```python
from build123d import *

# Parameters (mm, degrees)
SKETCH1_W                = 184.15
SKETCH1_H                = 184.15
BOSS_EXTRUDE1_DEPTH      = 3.175
CUT_EXTRUDE1_DEPTH       = 131.368453815
SKETCH3_R                = 6.477
SKETCH3_R_2              = 2.20345
CUT_EXTRUDE2_DEPTH       = 131.368453815
F_0_332_DIAMETER_HOLE1_D = 8.8392
FILLET1_R                = 12.7
FILLET2_R                = 101.6
CUT_EXTRUDE3_DEPTH       = 131.368453815
CUT_EXTRUDE3_DEPTH_BACK  = 131.368453815
SKETCH6_R                = 1.5367
SKETCH7_R                = 12.827
SKETCH7_R_2              = 3.2639
CUT_EXTRUDE4_DEPTH       = 131.368453815
SKETCH8_R                = 12.827
BOSS_EXTRUDE2_DEPTH      = 6.35


with BuildPart() as part:
    # Sketch1 → Boss-Extrude1 (new, symmetric)
    with BuildSketch(Plane(origin=(0, 0, 0), x_dir=(1, 0, 0), z_dir=(0, 1, 0))):
        Rectangle(SKETCH1_W, SKETCH1_H)
    extrude(amount=BOSS_EXTRUDE1_DEPTH, both=True)

    # Sketch2 → Cut-Extrude1 (cut, through all)
    with BuildSketch(Plane(origin=(0, 3.175, 0), x_dir=(1, 0, 0), z_dir=(0, 1, 0))):
        Polygon((92.075, -92.075), (92.075, 66.675), (-66.675, -92.075), align=None)
    extrude(amount=-CUT_EXTRUDE1_DEPTH, mode=Mode.SUBTRACT)

    # Sketch3 → Cut-Extrude2 (cut, through all)
    with BuildSketch(Plane(origin=(0, 3.175, 0), x_dir=(1, 0, 0), z_dir=(0, 1, 0))):
        with Locations(Location((-9.525, 9.525, 0), (0, 0, 270))):
            Circle(SKETCH3_R)
        with Locations(Location((-9.525, 19.84375, 0), (0, 0, 270))):
            Circle(SKETCH3_R_2)
        with Locations(Location((-9.525, -0.79375, 0), (0, 0, 270))):
            Circle(SKETCH3_R_2)
    extrude(amount=-CUT_EXTRUDE2_DEPTH, mode=Mode.SUBTRACT)

    # 0.332_ Diameter Hole1 (through all)
    with Locations(Plane(origin=(0, 3.175, 0), x_dir=(1, 0, 0), z_dir=(0, 1, 0))):
        with Locations((-73.025, -34.925), (-3.175, 73.025), (34.925, 73.025), (-73.025, 3.175)):
            Hole(F_0_332_DIAMETER_HOLE1_D / 2)

    # Fillet1
    fillet1_edges = [part.edges().sort_by_distance(p)[0] for p in [
        (-66.675, 0, 92.075),
        (92.075, 0, -66.675),
        (-92.075, 0, 92.075),
        (92.075, 0, -92.075),
    ]]
    fillet(fillet1_edges, radius=FILLET1_R)

    # Fillet2
    fillet2_edges = [part.edges().sort_by_distance(p)[0] for p in [
        (-92.075, 0, -92.075),
    ]]
    fillet(fillet2_edges, radius=FILLET2_R)

    # Sketch6 → Cut-Extrude3 (cut, two sides: drawn at the far end of the back side and taken through both)
    with BuildSketch(Plane.XZ.offset(3.175).offset(-CUT_EXTRUDE3_DEPTH_BACK)):
        with Locations(Location((73.025, -75.655256121, 0), (0, 0, 270))):
            Circle(SKETCH6_R)
        with Locations(Location((-23.731590206, -52.468409794, 0), (0, 0, 270))):
            Circle(SKETCH6_R)
        with Locations(Location((-75.655256121, 73.025, 0), (0, 0, 270))):
            Circle(SKETCH6_R)
        with Locations(Location((-52.468409794, -23.731590206, 0), (0, 0, 270))):
            Circle(SKETCH6_R)
    extrude(amount=CUT_EXTRUDE3_DEPTH + CUT_EXTRUDE3_DEPTH_BACK, mode=Mode.SUBTRACT)

    # Sketch7 → Cut-Extrude4 (cut, through all)
    with BuildSketch(Plane.XZ.offset(3.175)):
        with Locations(Location((-50.161792847, -50.161792847, 0), (0, 0, 270))):
            Circle(SKETCH7_R)
        with Locations(Location((-37.813940681, -62.509645014, 0), (0, 0, 270))):
            Circle(SKETCH7_R_2)
        with Locations(Location((-62.509645014, -37.813940681, 0), (0, 0, 270))):
            Circle(SKETCH7_R_2)
    extrude(amount=-CUT_EXTRUDE4_DEPTH, mode=Mode.SUBTRACT)

    # Sketch8 → Boss-Extrude2 (add)
    with BuildSketch(Plane.XZ.offset(3.175)):
        with Locations((-50.161792847, -50.161792847)):
            Circle(SKETCH8_R)
    extrude(amount=-BOSS_EXTRUDE2_DEPTH)


solid = part.part
```
The model under review builds one solid part; all positions refer to its coordinate system, in mm. Round coordinates to 2 decimals unless told otherwise and drop trailing zeros. Loops run counter-clockwise (first coordinate to the right, second up) from the corner with the lowest first, then second, coordinate; pieces in that order, holes last. Notation, with made-up numbers: (83.25, -4) - (121.25, -4) arc R13 cw to (121.25, 9) - close; hole circle Ø8 at (16.25, 17.5). An arc over 180 degrees is marked (long way). Write each question's results on one line, items separated by ' | '. Start each with the question number.
Q1. Draft analysis for pull direction Z (two halves, no side actions). For faces 1 (the cylindrical face through (-7.579, 0.044, -3.347)), 2 (the cylindrical face through (-7.34, 0.04, 0.51)), 3 (the cylindrical face through (91.08, -0.04, -67.01)), 4 (the cylindrical face through (88.26, -0.04, -88.45)), state which applies: pulls with the +Z half, pulls with the -Z half, needs draft (parallel to the pull), parting line crosses it, or undercut.
Q2. Take a section at C-C on x = 65. Give the boundary of the cut face in (y, z) (3 decimals).
Q3. Take a section at A-A on x = 33. Give the boundary of the cut face in (y, z) (3 decimals).
Q4. Take a section at B-B on y = 0.75. Give the number of separate pieces and of enclosed holes in the cut face, plus the area to 3 significant figures.
Q5. Take a section at D-D on x = -47.5. Give the boundary of the cut face in (y, z) (3 decimals).
Q6. Insertion check: P1, Ø1.8, axis at x = -75.66, z = 73.03, coming from the -Y side. The pin has a flat end and moves straight along its axis. Give the tip position at first contact, or say it passes through.
Q7. Wall thickness on line 1 along X through (y, z) = (0.75, -69); line 2 along Z through (x, y) = (-64.5, -1.75); line 3 along X through (y, z) = (0.25, -47.5): over which ranges is each line inside the solid? List them lowest first. Write a range as [from, to].
Data:
1) face 1: undercut | face 2: undercut | face 3: pulls with the +Z half | face 4: pulls with the -Z half
2) outline: (-3.175, -92.075) - (3.175, -92.075) - (3.175, -39.6) - (-3.175, -39.6) - close
3) outline: (-3.175, -92.075) - (3.175, -92.075) - (3.175, -77.003) - (-3.175, -77.003) - close; (-3.175, -69.047) - (3.175, -69.047) - (3.175, -7.6) - (-3.175, -7.6) - close
4) separate pieces: 1 | enclosed holes: 13 | area: 18,500 mm²
5) outline: (-3.175, -74.563) - (3.175, -74.563) - (3.175, 72.9) - (-3.175, 72.9) - close
6) P1: passes through
7) line 1: x = [-54.95, -5], [-1.35, 33.1], [36.75, 91.73] | line 2: z = [-60.07, -40.4], [-35.23, 89.67] | line 3: x = [-74.56, 72.9]
